Autodesk Inventor part; units mm, degrees
ref_plane "YZ Plane" through (0, 0, 0) normal (1, 0, 0) x (0, 1, 0)
ref_plane "XZ Plane" through (0, 0, 0) normal (0, 1, 0) x (-1, 0, 0)
ref_plane "XY Plane" through (0, 0, 0) normal (0, 0, 1) x (1, 0, 0)
sketch "Sketch1" plane through (0, 0, 0) normal (0, 0, 1) x (1, 0, 0)
  line L0 (0, 0) -> (100, 0) construction
  arc A0 (10.5, 0) -> (-3.0807, 10.0379) centre (0, 0) ccw construction
  arc A1 (89.5, 0) -> (95.0588, -9.2647) centre (100, 0) ccw construction
  arc A2 (95.0588, -9.2647) -> (60.7485, 1.3948) centre (50, -93.75) ccw
  arc A3 (103.0807, 10.0379) -> (64.7857, 17.3948) centre (50, -162.9167) ccw
  line L1 (35.2143, 17.3948) -> (64.7857, 17.3948)
  line L2 (39.2515, 1.3948) -> (60.7485, 1.3948)
  line L3 (50, 0) -> (50, 2) construction
  line L4 (50, 18) -> (50, 2) construction
  line L5 (35.2143, 17.3948) -> (39.2515, 1.3948) construction
  line L6 (0, 0) -> (37.2329, 9.3948) construction
  arc A4 (39.2515, 1.3948) -> (4.9412, -9.2647) centre (50, -93.75) ccw
  arc A5 (60.7485, 1.3948) -> (39.2515, 1.3948) centre (50, -93.75) ccw construction
  arc A6 (35.2143, 17.3948) -> (-3.0807, 10.0379) centre (50, -162.9167) ccw
  arc A7 (64.7857, 17.3948) -> (35.2143, 17.3948) centre (50, -162.9167) ccw construction
  arc A8 (4.9412, -9.2647) -> (10.5, 0) centre (0, 0) ccw construction
  arc A9 (-3.0807, 10.0379) -> (4.9412, -9.2647) centre (0, 0) ccw
  arc A10 (103.0807, 10.0379) -> (89.5, 0) centre (100, 0) ccw construction
  arc A11 (95.0588, -9.2647) -> (103.0807, 10.0379) centre (100, 0) ccw
  dimension "d0" = 100
  dimension "d1" = 21
  dimension "d2" = 2
  dimension "d3" = 16
  dimension "d30" = 16
  dimension "d31" = 38.3998
extrude "Extrusion1" add sketch "Sketch1" along normal blind 2
sketch "Sketch2" plane through (0, 0, 2) normal (0, 0, 1) x (1, 0, 0)
  line L0 (64.7857, 17.3948) -> (35.2143, 17.3948) construction
  line L1 (39.2515, 1.3948) -> (60.7485, 1.3948) construction
  line L2 (50, 17.3948) -> (50, 1.3948) construction
  line L3 (41, 9.3948) -> (59, 9.3948) construction
  line L4 (46, 6.8448) -> (54, 6.8448)
  line L5 (54, 6.8448) -> (54, 11.9448)
  line L6 (54, 11.9448) -> (46, 11.9448)
  line L7 (46, 11.9448) -> (46, 6.8448)
  line L8 (46, 6.8448) -> (54, 11.9448) construction
  line L9 (54, 6.8448) -> (46, 11.9448) construction
  point P0 (0, 0)
  point P1 (50, 9.3948)
  dimension "d7" = 18
  dimension "d8" = 5.1
  dimension "d9" = 8
extrude "Extrusion2" cut sketch "Sketch2" against normal through all
hole "Hole1" at (41, 9.3948, 2) at (59, 9.3948, 2) direction (0, 0, -1) diameter 2.6 end through all
sketch "Sketch3" plane through (0, 0, 2) normal (0, 0, 1) x (1, 0, 0)
  line L0 (46, 11.9448) -> (54, 11.9448) construction
  line L1 (46, 6.8448) -> (46, 11.9448) construction
  line L2 (54, 6.8448) -> (46, 6.8448) construction
  line L3 (54, 11.9448) -> (54, 6.8448) construction
  line L4 (53.2929, 11.2377) -> (46.7071, 11.2377) construction
  line L5 (46.7071, 11.2377) -> (46.7071, 7.5519) construction
  line L6 (46.7071, 7.5519) -> (53.2929, 7.5519) construction
  line L7 (53.2929, 7.5519) -> (53.2929, 11.2377) construction
  circle A0 centre (46.7071, 11.2377) radius 1
  circle A1 centre (46.7071, 7.5519) radius 1
  circle A2 centre (53.2929, 7.5519) radius 1
  circle A3 centre (53.2929, 11.2377) radius 1
  point P0 (0, 0)
  dimension "d19" = 2
extrude "Extrusion3" cut sketch "Sketch3" against normal through all
sketch "Sketch4" plane through (0, 0, 2) normal (0, 0, 1) x (1, 0, 0)
  arc A0 (95.0588, -9.2647) -> (103.0807, 10.0379) centre (100, 0) ccw construction
  point P0 (0, 0)
  point P1 (0, 0)
hole "Hole2" at (0, 0, 2) at (100, 0, 2) direction (0, 0, -1) diameter 8 end through all
sketch "Sketch5" plane through (0, 0, 2) normal (0, 0, 1) x (1, 0, 0)
  circle A0 centre (0, 0) radius 8 construction
  circle A1 centre (100, 0) radius 4 construction
  circle A2 centre (100, 0) radius 8 construction
  line L0 (-8, 0) -> (0, 0) construction
  line L1 (100, 0) -> (108, 0) construction
  point P0 (-5.6569, -5.6569)
  point P1 (0, -8)
  point P2 (5.6569, -5.6569)
  point P3 (8, 0)
  point P4 (5.6569, 5.6569)
  point P5 (0, 8)
  point P6 (-5.6569, 5.6569)
  point P7 (105.6569, 5.6569)
  point P8 (100, 8)
  point P9 (94.3431, 5.6569)
  point P10 (92, 0)
  point P11 (94.3431, -5.6569)
  point P12 (100, -8)
  point P13 (105.6569, -5.6569)
  dimension "d36" = 16
  dimension "d34" = 360
  dimension "d39" = 360
hole "Hole3" at (-8, 0, 2) at (-5.6569, -5.6569, 2) at (0, -8, 2) at (5.6569, -5.6569, 2) at (8, 0, 2) at (5.6569, 5.6569, 2) at (0, 8, 2) at (-5.6569, 5.6569, 2) at (108, 0, 2) at (105.6569, 5.6569, 2) at (100, 8, 2) at (94.3431, 5.6569, 2) at (92, 0, 2) at (94.3431, -5.6569, 2) at (100, -8, 2) at (105.6569, -5.6569, 2) direction (0, 0, -1) diameter 2.2 end through all
fillet "Fillet1" radius 3 4 edges at (35.2143, 17.3948, 1) (64.7857, 17.3948, 1) (60.7485, 1.3948, 1) (39.2515, 1.3948, 1)
sketch "Sketch6" plane through (0, 0, 2) normal (0, 0, 1) x (1, 0, 0)
  arc A0 (64.9097, 17.3846) -> (64.6624, 17.3948) centre (64.6624, 14.3948) ccw
  line L0 (64.6624, 17.3948) -> (35.3376, 17.3948)
  arc A1 (35.3376, 17.3948) -> (35.0903, 17.3846) centre (35.3376, 14.3948) ccw
  arc A2 (35.0903, 17.3846) -> (-3.0807, 10.0379) centre (50, -162.9167) ccw
  arc A3 (-3.0807, 10.0379) -> (4.9412, -9.2647) centre (0, 0) ccw
  arc A4 (39.0796, 1.3752) -> (4.9412, -9.2647) centre (50, -93.75) ccw
  arc A5 (39.4217, 1.3948) -> (39.0796, 1.3752) centre (39.4217, -1.6052) ccw
  line L1 (39.4217, 1.3948) -> (60.5783, 1.3948)
  arc A6 (60.9204, 1.3752) -> (60.5783, 1.3948) centre (60.5783, -1.6052) ccw
  arc A7 (95.0588, -9.2647) -> (60.9204, 1.3752) centre (50, -93.75) ccw
  arc A8 (95.0588, -9.2647) -> (103.0807, 10.0379) centre (100, 0) ccw
  arc A9 (103.0807, 10.0379) -> (64.9097, 17.3846) centre (50, -162.9167) ccw
  circle A10 centre (100, -8) radius 1.1
  circle A11 centre (92, 0) radius 1.1
  circle A12 centre (100, 8) radius 1.1
  circle A13 centre (108, 0) radius 1.1
  circle A14 centre (0, 8) radius 1.1
  circle A15 centre (8, 0) radius 1.1
  circle A16 centre (0, -8) radius 1.1
  circle A17 centre (-8, 0) radius 1.1
  circle A18 centre (-5.6569, -5.6569) radius 1.1
  circle A19 centre (5.6569, -5.6569) radius 1.1
  circle A20 centre (5.6569, 5.6569) radius 1.1
  circle A21 centre (-5.6569, 5.6569) radius 1.1
  circle A22 centre (105.6569, 5.6569) radius 1.1
  circle A23 centre (94.3431, 5.6569) radius 1.1
  circle A24 centre (94.3431, -5.6569) radius 1.1
  circle A25 centre (105.6569, -5.6569) radius 1.1
  circle A26 centre (0, 0) radius 4
  circle A27 centre (100, 0) radius 4
  arc A28 (52.5858, 6.8448) -> (54, 8.259) centre (53.2929, 7.5519) ccw
  line L2 (52.5858, 6.8448) -> (47.4142, 6.8448)
  arc A29 (46, 8.259) -> (47.4142, 6.8448) centre (46.7071, 7.5519) ccw
  line L3 (46, 8.259) -> (46, 10.5306)
  arc A30 (47.4142, 11.9448) -> (46, 10.5306) centre (46.7071, 11.2377) ccw
  line L4 (47.4142, 11.9448) -> (52.5858, 11.9448)
  arc A31 (54, 10.5306) -> (52.5858, 11.9448) centre (53.2929, 11.2377) ccw
  line L5 (54, 10.5306) -> (54, 8.259)
  circle A32 centre (41, 9.3948) radius 1.3
  circle A33 centre (59, 9.3948) radius 1.3
properties part number "16_012_FEMUR_FRAME_DRIVER_R1" material "Aluminum 6061"
Geometry: final body of the model. Coordinates: model frame, mm. A direction names the side the tool comes from. Coordinates: 2 decimals unless noted, no trailing zeros. Order: outer loops, then holes, each group sorted by start corner. A loop starts at its lowest first (then second) coordinate and runs counter-clockwise, first axis right, second up. Notation, with made-up numbers: (5.25, -17) -> (50.25, -17) arc R30 cw to (50.25, 13) -> close; hole circle Ø8 at (55.25, 57.25). An arc over 180 degrees is marked (long way). Answer in a Markdown table with one row per item.
Item 1: Access query for faces 1 (the flat face through (49, 4, 2)), 2 (the flat face through (46, 9, 1)). Directions: +Z, -Z, +X, -X, +Y, -Y. A direction counts if a zero-diameter tool reaches every point of the face in a straight line with its end or side. Return the directions, or none.
Return value:
| item | result |
|---|---|
| face 1 | +Z, +X, -X, +Y, -Y |
| face 2 | +Z, -Z |
Item 2: Ray query, L1, parallel to X at y = -7.25, z = 0.85; L2, parallel to Y at x = 48.5, z = 1; L3, parallel to X at y = 8, z = 0.7. Return the intervals inside material, ascending.
Return value:
| item | result |
|---|---|
| L1 | x = -7.6 to -0.8, 0.8 to 8.94, 91.06 to 99.2, 100.8 to 107.6 |
| L2 | y = 1.39 to 6.84, 11.94 to 17.39 |
| L3 | x = -6.8 to -1.1, 1.1 to 45.81, 54.19 to 98.9, 101.1 to 106.8 |
Item 3: Draft query along X for faces 3 (the cylindrical face through (106.633, -6.164, 0.986)), 4 (the flat face through (50, 17.395, 1)). Return one class per face: released by +X, released by -X, zero draft, split by the parting line, or undercut.
Return value:
| item | result |
|---|---|
| face 3 | undercut |
| face 4 | zero draft |
Item 4: Contact query for flat-ended pins moving along their axis: P1, Ø2, axis at x = 105.66, y = 5.66, coming from the +Z side; P2, Ø1, axis at y = 7.5, z = 1.5, coming from the -X side. Output: stop coordinate, or through.
Return value:
| item | result |
|---|---|
| P1 | passes through |
| P2 | stops at x = -7.83 |
Item 5: Section D-D on x = -8. Output: boundary loops of the cut face in (y, z).
Return value:
| item | result |
|---|---|
| outline | (-6.8, 0) -> (-1.1, 0) -> (-1.1, 2) -> (-6.8, 2) -> close; (1.1, 0) -> (6.8, 0) -> (6.8, 2) -> (1.1, 2) -> close |
Item 6: Section B-B on x = 100. Output: boundary loops of the cut face in (y, z).
Return value:
| item | result |
|---|---|
| outline | (-10.5, 0) -> (-9.1, 0) -> (-9.1, 2) -> (-10.5, 2) -> close; (-6.9, 0) -> (-4, 0) -> (-4, 2) -> (-6.9, 2) -> close; (4, 0) -> (6.9, 0) -> (6.9, 2) -> (4, 2) -> close; (9.1, 0) -> (10.95, 0) -> (10.95, 2) -> (9.1, 2) -> close |
Item 7: Section C-C on y = 15.75. Output: boundary loops of the cut face in (x, z), plus the area to 3 significant figures.
Return value:
| item | result |
|---|---|
| outline | (21.56, 0) -> (78.44, 0) -> (78.44, 2) -> (21.56, 2) -> close |
| area | 114 mm² |
Item 8: Section A-A on x = 41. Output: boundary loops of the cut face in (y, z).
Return value:
| item | result |
|---|---|
| outline | (1.39, 0) -> (8.09, 0) -> (8.09, 2) -> (1.39, 2) -> close; (10.69, 0) -> (17.39, 0) -> (17.39, 2) -> (10.69, 2) -> close |
